Could you check a few things on this drawing? It's one solid part, dimensions in mm from its lowest x, y, z. A direction names the side the tool comes from. Give positions to 0.01 mm unless a question says otherwise; leave off trailing zeros. Loops run counter-clockwise (first coordinate to the right, second up) from the corner with the lowest first, then second, coordinate; pieces in that order, holes last. Notation, with made-up numbers: M -3.75,89.5 L 50.25,89.5 A31 cw 50.25,118.5 Z; hole C 40.5,55 d6. An arc over 180 degrees is marked long. Return JSON: item names as keys, results as strings. Group by question number.
1. For pin 1 (4.5 mm diameter, centred on x = 12.7, z = 11.11, fed in from -Y); pin 2 (12 mm diameter, centred on y = 27.5, z = 35.5, fed in from -X); pin 3 (6 mm diameter, centred on y = 23.5, z = 34, fed in from +X) (1 decimal); pin 4 (19 mm diameter, centred on x = 22, z = 25, fed in from +Y) (1 decimal), each with a flat end and sliding along its axis, tell me the tip position at first contact or that it passes through.
2. If we section it at D-D (x = 30.5): Write out the boundary of the cut face in (y, z) (1 decimal).
3. Please list where these lines run through material, in increasing order: line 1 (Z direction, x = 12.7, y = 2.6) (1 decimal); line 2 (Z direction, x = 12, y = 2) (1 decimal); line 3 (X direction, y = 41, z = 43) (1 decimal).
4. If we section it at A-A (y = 38.1): Write out the boundary of the cut face in (x, z) (1 decimal), plus the area to 3 significant figures.
5. If we section it at C-C (z = 9.5): State how many separate pieces and enclosed holes the cut face has, plus the area to 3 significant figures.
6. If we mould it in two halves opening along Y, with no side actions, what happens to the marked faces 1, 2 and 3? For each: +Y half, -Y half, draft (parallel to the pull), parting line (faces both ways), or undercut.
7. For the marked faces 4 and 5, which set-ups out of +Z, -Z, +X, -X, +Y, -Y let a thin tool reach every point of the face, with its end or its side?
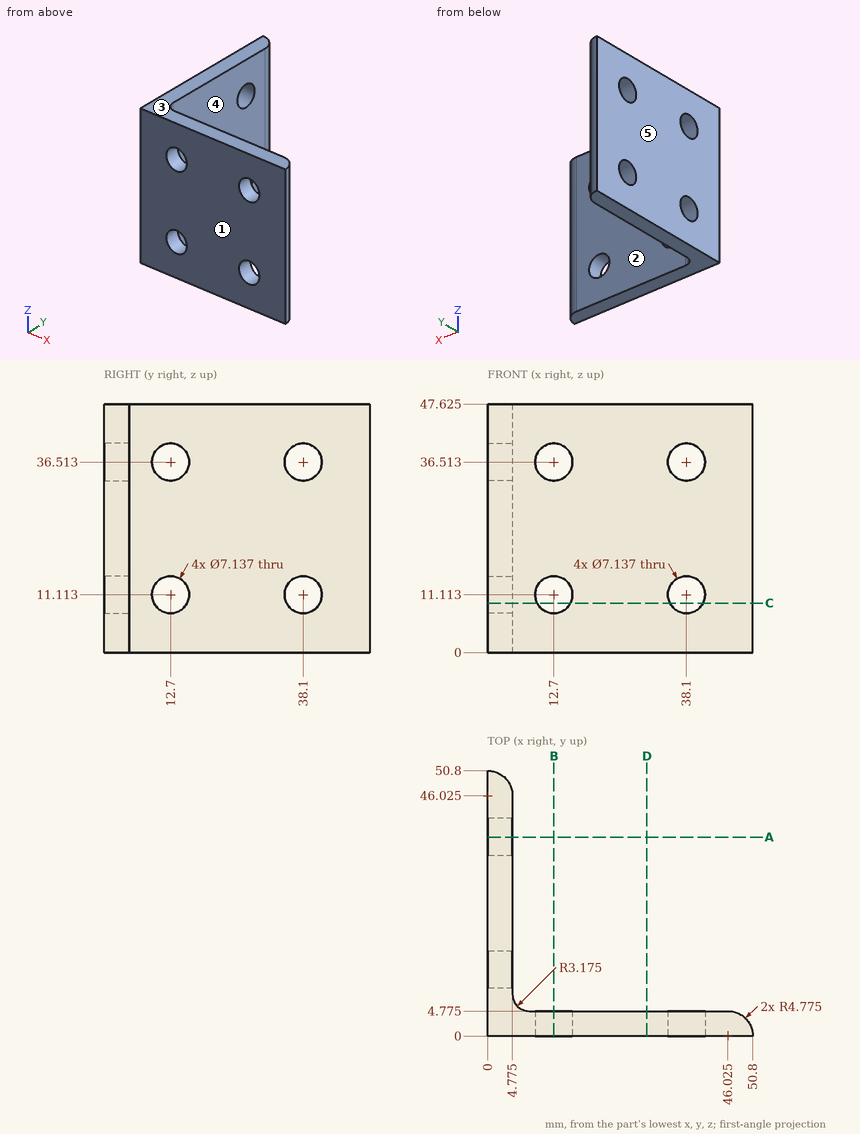
Answer:
{
 "1": {"pin 1": "passes through", "pin 2": "stops at x = 0", "pin 3": "stops at x = 4.8", "pin 4": "stops at y = 4.8"},
 "2": {"outline": "M 0,0 L 4.8,0 L 4.8,47.6 L 0,47.6 Z"},
 "3": {"line 1": "z = 0 to 7.5, 14.7 to 32.9, 40.1 to 47.6", "line 2": "z = 0 to 7.6, 14.6 to 33, 40 to 47.6", "line 3": "x = 0 to 4.8"},
 "4": {"outline": "M 0,0 L 4.8,0 L 4.8,7.5 L 0,7.5 Z; M 0,14.7 L 4.8,14.7 L 4.8,32.9 L 0,32.9 Z; M 0,40.1 L 4.8,40.1 L 4.8,47.6 L 0,47.6 Z", "area": "159 mm²"},
 "5": {"separate pieces": "5", "enclosed holes": "0", "area": "333 mm²"},
 "6": {"face 1": "-Y half", "face 2": "+Y half", "face 3": "draft"},
 "7": {"face 4": "+Z, -Z, +X, +Y", "face 5": "+Z, -Z, -X, +Y, -Y"}
}
